from build123d import *

# Parameters (mm, degrees)
F1_DEPTH = 25.4
F2_DEPTH = 50.8
F0_W     = 101.6
F0_H     = 177.8
F3_DEPTH = 6.35
F4_R     = 6.34999
F5_SIZE  = 12.7
F6_SIZE  = 12.7


# Not quite as in the source:
# - a fillet or chamfer is up to 0.001 mm smaller than in the source, because OpenCascade refuses the exact size
# - a length typed as a fraction of an inch, garbled in the dataset ("3 / 203.2 mm" for 3/8 in), is restored


with BuildPart() as f1:
    # F0 (on Top) → F1 (new body)
    with BuildSketch(Plane.XY):
        with BuildLine():
            Line((44.7456893295, 103.9061718148), (6.6456893295, 103.9061718148))
            Line((6.6456893295, 103.9061718148), (6.6456893295, 78.5061718148))
            ThreePointArc((6.6456893295, 78.5061718148), (2.9259454506, 69.5259156938), (-6.0543106705, 65.8061718148))
            Line((-6.0543106705, 65.8061718148), (-31.4543106705, 65.8061718148))
            Line((-31.4543106705, 65.8061718148), (-31.4543106705, -48.4938281852))
            Line((-31.4543106705, -48.4938281852), (6.6456893295, -48.4938281852))
            Line((6.6456893295, -48.4938281852), (6.6456893295, -23.0938281852))
            ThreePointArc((6.6456893295, -23.0938281852), (10.3654332084, -14.1135720641), (19.3456893295, -10.3938281852))
            Line((19.3456893295, -10.3938281852), (44.7456893295, -10.3938281852))
            Line((44.7456893295, -10.3938281852), (44.7456893295, 103.9061718148))
        make_face()
    extrude(amount=F1_DEPTH)

    # F0 (on Top) → F2 (join)
    with BuildSketch(Plane.XY):
        with BuildLine():
            Line((6.6456893295, 103.9061718148), (-31.4543106705, 103.9061718148))
            Line((-31.4543106705, 103.9061718148), (-31.4543106705, 65.8061718148))
            Line((-31.4543106705, 65.8061718148), (-6.0543106705, 65.8061718148))
            ThreePointArc((-6.0543106705, 65.8061718148), (2.9259454506, 69.5259156938), (6.6456893295, 78.5061718148))
            Line((6.6456893295, 78.5061718148), (6.6456893295, 103.9061718148))
        make_face()
        with BuildLine():
            Line((44.7456893295, -48.4938281852), (44.7456893295, -10.3938281852))
            Line((44.7456893295, -10.3938281852), (19.3456893295, -10.3938281852))
            ThreePointArc((19.3456893295, -10.3938281852), (10.3654332084, -14.1135720641), (6.6456893295, -23.0938281852))
            Line((6.6456893295, -23.0938281852), (6.6456893295, -48.4938281852))
            Line((6.6456893295, -48.4938281852), (44.7456893295, -48.4938281852))
        make_face()
    extrude(amount=F2_DEPTH)

    # F0 (on Top) → F3 (join)
    with BuildSketch(Plane.XY):
        with Locations((6.6456893295, 27.7061718148)):
            Rectangle(F0_W, F0_H)
        Polygon((-31.4543106705, 65.8061718148), (-31.4543106705, 103.9061718148), (6.6456893295, 103.9061718148), (44.7456893295, 103.9061718148), (44.7456893295, -10.3938281852), (44.7456893295, -48.4938281852), (6.6456893295, -48.4938281852), (-31.4543106705, -48.4938281852), align=None, mode=Mode.SUBTRACT)
    extrude(amount=F3_DEPTH)

    # F4 (radius 6.35 in the source; OpenCascade refuses exactly that, so slightly less here)
    f4_edges = [f1.edges().sort_by_distance(p)[0] for p in [
        (6.645689, -61.193828, 6.35),
        (-44.154311, 27.706172, 6.35),
        (6.645689, 116.606172, 6.35),
        (57.445689, 27.706172, 6.35),
    ]]
    fillet(f4_edges, radius=F4_R)

    # F5
    f5_edges = [f1.edges().sort_by_distance(p)[0] for p in [
        (-12.404311, -48.493828, 25.4),
        (-31.454311, 8.656172, 25.4),
        (44.745689, 46.756172, 25.4),
        (25.695689, 103.906172, 25.4),
    ]]
    chamfer(f5_edges, length=F5_SIZE)

    # F6
    f6_edges = [f1.edges().sort_by_distance(p)[0] for p in [
        (44.745689, -29.443828, 50.8),
        (25.695689, -48.493828, 50.8),
        (-31.454311, 84.856172, 50.8),
        (-12.404311, 103.906172, 50.8),
    ]]
    chamfer(f6_edges, length=F6_SIZE)


solid = f1.part
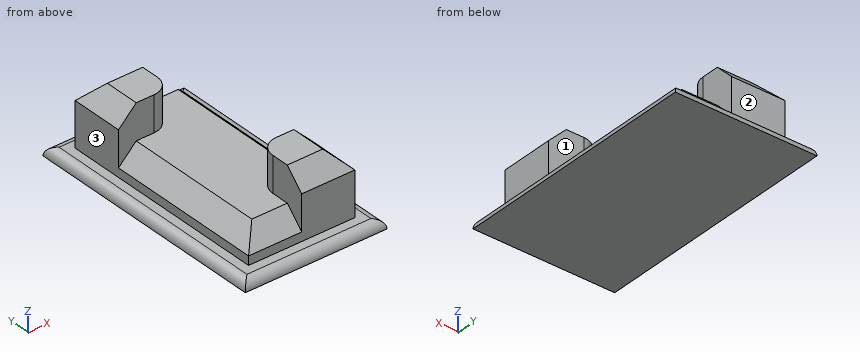
Input: part model. Units: mm. Frame: model coordinates. Face numbers are marked on the shaded views. A direction names the side the tool comes from. Coordinates: 2 decimals unless noted, no trailing zeros. Loops run counter-clockwise (first coordinate to the right, second up) from the corner with the lowest first, then second, coordinate; pieces in that order, holes last.
Q1. Cut plane A-A (z = 31). Output: boundary loops of the cut face in (x, y).
Q2. Material intervals for line 1 (Y direction, x = 20.5, z = 9.5); line 2 (Z direction, x = 30, y = 32.5); line 3 (Z direction, x = 2, y = -50), sorted ascending.
Q3. Set-up query: the marked faces 1, 2 and 3. Return all of +Z, -Z, +X, -X, +Y, -Y with unobstructed straight access to the full face (end or side cutting, diameter ignored); none if empty.
Q4. Contact query for flat-ended pins moving along their axis: pin 1 (3 mm diameter, centred on x = 10.5, z = 24, fed in from +Y); pin 2 (20.5 mm diameter, centred on y = -32.5, z = 39.5, fed in from -X); pin 3 (9.5 mm diameter, centred on x = 18, z = 25, fed in from +Y); pin 4 (4 mm diameter, centred on x = -33.5, z = 37.5, fed in from +Y) (3 decimals). Output: stop coordinate, or through.
Q5. Cut plane D-D (z = 11). Output: boundary loops of the cut face in (x, y), then the cut area to 3 significant figures.
Working result:
1. outline: (-31.45, 65.81) - (-6.05, 65.81) arc R12.7 ccw to (6.65, 78.51) - (6.65, 103.91) - (-31.45, 103.91) - close; (6.65, -48.49) - (44.75, -48.49) - (44.75, -10.39) - (19.35, -10.39) arc R12.7 ccw to (6.65, -23.09) - close
2. line 1: y = -48.49 to 103.91
2. line 2: z = 0 to 25.4
2. line 3: z = 0 to 6.35
3. face 1: +Z, +X, +Y
3. face 2: +Z, +X, -X, +Y
3. face 3: +Z, -X, +Y, -Y
4. pin 1: stops at y = 94.11
4. pin 2: stops at x = 6.65
4. pin 3: stops at y = 96.36
4. pin 4: passes through
5. outline: (-31.45, -48.49) - (44.75, -48.49) - (44.75, 103.91) - (-31.45, 103.91) - close
5. area: 11,600 mm2
